```python
from build123d import *

# Parameters (mm, degrees)
F1_DEPTH = 3.175


with BuildPart() as f1:
    # F0 (on Front) → F1 (new body)
    with BuildSketch(Plane.XZ):
        Polygon((-1.2503195478, 0), (0, 0), (0, 1.9634975899), (-16.2488400529, 1.9634975899), (-12.7, 0), align=None)
        Polygon((0, 1.9634975899), (0, 0), (1.2503195478, 0), (12.7, 0), (16.2488400529, 1.9634975899), align=None)
        with BuildLine():
            Line((16.2488400529, 1.9634975899), (12.7, 0))
            Line((12.7, 0), (5.273375106, -10.9961956262))
            ThreePointArc((5.273375106, -10.9961956262), (6.1114552938, -11.6331804071), (6.8732481888, -12.3596785818))
            Line((6.8732481888, -12.3596785818), (16.2488400529, 1.9634975899))
        make_face()
        with BuildLine():
            Line((-5.273375106, -10.9961956262), (-12.7, 0))
            Line((-12.7, 0), (-16.2488400529, 1.9634975899))
            Line((-16.2488400529, 1.9634975899), (-6.8732481888, -12.3596785818))
            ThreePointArc((-6.8732481888, -12.3596785818), (-6.1114552938, -11.6331804071), (-5.273375106, -10.9961956262))
        make_face()
        with BuildLine():
            Line((1.2503195478, 0), (0, 0))
            Line((0, 0), (-1.2503195478, 0))
            Line((-1.2503195478, 0), (-1.2503195478, -9.4655629921))
            ThreePointArc((-1.2503195478, -9.4655629921), (0, -9.3822341022), (1.2503195478, -9.4655629921))
            Line((1.2503195478, -9.4655629921), (1.2503195478, 0))
        make_face()
        with BuildLine():
            Line((1.2503195478, -11.6856056581), (1.2503195478, -9.4655629921))
            ThreePointArc((1.2503195478, -9.4655629921), (0, -9.3822341022), (-1.2503195478, -9.4655629921))
            Line((-1.2503195478, -9.4655629921), (-1.2503195478, -11.6856056581))
            ThreePointArc((-1.2503195478, -11.6856056581), (0, -11.5766356799), (1.2503195478, -11.6856056581))
        make_face()
        with BuildLine():
            Line((-1.2503195478, -11.6856056581), (-1.2503195478, -9.4655629921))
            ThreePointArc((-1.2503195478, -9.4655629921), (-3.3504263981, -9.9980615076), (-5.273375106, -10.9961956262))
            Line((-5.273375106, -10.9961956262), (-4.0451906764, -12.8147008617))
            ThreePointArc((-4.0451906764, -12.8147008617), (-2.7072718978, -12.1028302128), (-1.2503195478, -11.6856056581))
        make_face()
        with BuildLine():
            Line((-4.0451906764, -12.8147008617), (-5.273375106, -10.9961956262))
            ThreePointArc((-5.273375106, -10.9961956262), (-6.1114552938, -11.6331804071), (-6.8732481888, -12.3596785818))
            Line((-6.8732481888, -12.3596785818), (-5.6253009067, -14.2661788895))
            ThreePointArc((-5.6253009067, -14.2661788895), (-4.8894068128, -13.4814790218), (-4.0451906764, -12.8147008617))
        make_face()
        with BuildLine():
            Line((-5.6253009067, -14.2661788895), (-6.8732481888, -12.3596785818))
            ThreePointArc((-6.8732481888, -12.3596785818), (-3.4651004367, -27.5658350731), (9.4219584409, -18.804192543))
            ThreePointArc((9.4219584409, -18.804192543), (8.7616425301, -15.3390921063), (6.8732481888, -12.3596785818))
            Line((6.8732481888, -12.3596785818), (5.6253009067, -14.2661788895))
            ThreePointArc((5.6253009067, -14.2661788895), (6.8152314849, -16.3979095137), (7.2275568631, -18.804192543))
            ThreePointArc((7.2275568631, -18.804192543), (-2.4062830293, -25.6194240279), (-5.6253009067, -14.2661788895))
        make_face()
        with BuildLine():
            Line((-1.2503195478, -16.9529130534), (-4.0451906764, -12.8147008617))
            ThreePointArc((-4.0451906764, -12.8147008617), (-4.8894068128, -13.4814790218), (-5.6253009067, -14.2661788895))
            Line((-5.6253009067, -14.2661788895), (0, -22.8600017726))
            Line((0, -22.8600017726), (0, -18.804192543))
            Line((0, -18.804192543), (-1.2503195478, -16.9529130534))
        make_face()
        with BuildLine():
            ThreePointArc((5.6253009067, -14.2661788895), (4.8894068128, -13.4814790218), (4.0451906764, -12.8147008617))
            Line((4.0451906764, -12.8147008617), (1.2503195478, -16.9529130534))
            Line((1.2503195478, -16.9529130534), (0, -18.804192543))
            Line((0, -18.804192543), (0, -22.8600017726))
            Line((0, -22.8600017726), (5.6253009067, -14.2661788895))
        make_face()
        with BuildLine():
            ThreePointArc((5.273375106, -10.9961956262), (3.3504263981, -9.9980615076), (1.2503195478, -9.4655629921))
            Line((1.2503195478, -9.4655629921), (1.2503195478, -11.6856056581))
            ThreePointArc((1.2503195478, -11.6856056581), (2.7072718978, -12.1028302128), (4.0451906764, -12.8147008617))
            Line((4.0451906764, -12.8147008617), (5.273375106, -10.9961956262))
        make_face()
        with BuildLine():
            ThreePointArc((6.8732481888, -12.3596785818), (6.1114552938, -11.6331804071), (5.273375106, -10.9961956262))
            Line((5.273375106, -10.9961956262), (4.0451906764, -12.8147008617))
            ThreePointArc((4.0451906764, -12.8147008617), (4.8894068128, -13.4814790218), (5.6253009067, -14.2661788895))
            Line((5.6253009067, -14.2661788895), (6.8732481888, -12.3596785818))
        make_face()
    extrude(amount=F1_DEPTH)


solid = f1.part
```
Work out the finished part from the listing and answer in its coordinate system (mm). A direction names the side the tool comes from. Give positions to 0.01 mm unless a question says otherwise; leave off trailing zeros. Order: outer loops, then holes, each group sorted by start corner. A loop starts at its lowest first (then second) coordinate and runs counter-clockwise, first axis right, second up.
1. Straight lines are drawn through the part: L1, parallel to Z at x = 6, y = -1.25; L2, parallel to X at y = -2.3, z = -22.5; L3, parallel to X at y = -0.3, z = -15.5. For each, find the intervals that lie inside material, in ascending order.
Result sheet:
L1: z = -26.07 to -22.83, -14.77 to -9.92, 0 to 1.96
L2: x = -8.67 to -6.21, -0.24 to 0.24, 6.21 to 8.67
L3: x = -8.82 to -6.43, -4.82 to -2.23, 2.23 to 4.82, 6.43 to 8.82
2. Section A-A, the plane x = 3 is taken. Determine the outline of the cut face in (y, z) (1 decimal).
Result sheet:
outline: (-3.2, -27.7) - (0, -27.7) - (0, -25.4) - (-3.2, -25.4) - close; (-3.2, -18.3) - (0, -18.3) - (0, -14.4) - (-3.2, -14.4) - close; (-3.2, -12.2) - (0, -12.2) - (0, -9.9) - (-3.2, -9.9) - close; (-3.2, 0) - (0, 0) - (0, 2) - (-3.2, 2) - close
3. Section B-B, the plane y = -2.8 is taken. Determine the outline of the cut face in (x, z), and give its area (3 significant figures).
Result sheet:
outline: (-16.25, 1.96) - (-6.87, -12.36) arc R9.42 ccw (long way) to (6.87, -12.36) - (16.25, 1.96) - close; hole (-12.7, 0) - (-5.27, -11) arc R9.42 cw to (-1.25, -9.47) - (-1.25, 0) - close; hole (-5.63, -14.27) arc R7.23 ccw (long way) to (5.63, -14.27) - (0, -22.86) - close; hole (-4.05, -12.81) - (0, -18.8) - (4.05, -12.81) arc R7.23 ccw to start; hole (1.25, -9.47) arc R9.42 cw to (5.27, -11) - (12.7, 0) - (1.25, 0) - close
area: 294 mm2
4. Section D-D, the plane z = -6 is taken. Determine the outline of the cut face in (x, y) (3 decimals), and give its area (3 significant figures).
Result sheet:
outline: (-11.036, -3.175) - (-8.648, -3.175) - (-8.648, 0) - (-11.036, 0) - close; (-1.25, -3.175) - (1.25, -3.175) - (1.25, 0) - (-1.25, 0) - close; (8.648, -3.175) - (11.036, -3.175) - (11.036, 0) - (8.648, 0) - close
area: 23.1 mm2
5. The mould has two halves that part along Z. Classify faces 1 (the flat face through (1.25, -2, -5)), 2 (the flat face through (0, 0, -11)), 3 (the flat face through (0, -2, 1.963)): released by +Z, released by -Z, zero draft, split by the parting line, or undercut.
Result sheet:
face 1: undercut
face 2: zero draft
face 3: released by +Z
6. For faces 4 (the flat face through (0, -3.175, -11)), 5 (the flat face through (11.495, -1.565, -5.298)), 6 (the flat face through (-2.852, -1.565, -18.503)), 7 (the flat face through (-11.627, -1.565, -5.098)), determine the directions among +Z, -Z, +X, -X, +Y, -Y from which every point of the face is accessible in a straight line to the end or side of a thin tool.
Result sheet:
face 4: +Z, -Z, +X, -X, -Y
face 5: +X, +Y, -Y
face 6: +Y, -Y
face 7: -X, +Y, -Y
7. Section C-C, the plane z = -15 is taken. Determine the outline of the cut face in (x, y) (3 decimals).
Result sheet:
outline: (-8.62, -3.175) - (-6.145, -3.175) - (-6.145, 0) - (-8.62, 0) - close; (-5.145, -3.175) - (-2.569, -3.175) - (-2.569, 0) - (-5.145, 0) - close; (2.569, -3.175) - (5.145, -3.175) - (5.145, 0) - (2.569, 0) - close; (6.145, -3.175) - (8.62, -3.175) - (8.62, 0) - (6.145, 0) - close
8. Each of these flat-tipped pins is pushed along its axis until it touches: P1, Ø1, axis at x = 5, y = -1.5, coming from the -Z side; P2, Ø1, axis at y = -2, z = -5.5, coming from the +X side. Where does it stop, or does it pass through?
Result sheet:
P1: stops at z = -27.08
P2: stops at x = 11.69
